Geometry check sheet. Reference: the model listing, model coordinates, mm. A direction names the side the tool comes from. Give positions to 0.01 mm unless a question says otherwise; leave off trailing zeros. Write each loop counter-clockwise with the first axis right and the second up, starting at its lowest first coordinate (ties: lowest second). Pieces come first, ordered by that corner, then holes. Notation, with made-up numbers: (87, 3.5) - (132, 3.5) arc R22 ccw to (132, 28.5) - close; hole circle Ø5 at (5, -21). An arc over 180 degrees is marked (long way). One line per question, with ' | ' between items. Start each with the question number.
Q1. Section check D-D on y = 30. Record the boundary of the cut face in (x, z).
Q2. Release check for a two-part mould opening along Y. For faces 6 (the face through (104, 28, 17)), 7 (the face through (105.014, 31.636, 17.215)), 8 (the face through (1.141, 1.203, 5.916)), 9 (the face through (64, 106, 11)) record: +Y half, -Y half, draft (parallel to the pull), parting line (faces both ways), or undercut.
Q3. Thickness scan on L1, parallel to Y at x = 105.05, z = 17; L2, parallel to Y at x = 98.5, z = 11; L3, parallel to X at y = 105.1, z = 17. Record the ranges inside material, lowest first. Write a range as [from, to].
Q4. Gauge pin test, flat ends, axial feed: P1, Ø5, axis at x = 14.5, y = 45, coming from the +Z side; P2, Ø9.5, axis at x = 86.5, z = 7, coming from the +Y side; P3, Ø1.6, axis at x = 103, y = 82.5, coming from the +Z side. Record the tip position at first contact, or that the pin passes through.
Q5. Section check A-A on x = 64. Record the boundary of the cut face in (y, z), and give its area (3 significant figures).
Q6. Section check C-C on z = 17. Record the boundary of the cut face in (x, y), and give its area (3 significant figures).
Q7. Set-up check for faces 1 (the face through (51, 53, 2)), 2 (the face through (102.797, 1.141, 5.916)), 3 (the face through (62, 104, 17)), 4 (the face through (62.536, 105.014, 17.761)), 5 (the face through (28, 104, 6)): record each of +Z, -Z, +X, -X, +Y, -Y from which the full face is reachable in a straight line by a thin tool's end or side.
Q8. Section check B-B on x = 26.5. Record the boundary of the cut face in (y, z), and give its area (3 significant figures).
```python
from build123d import *

# Parameters (mm, degrees)
EXTRUDE_2_DEPTH     = 2
EXTRUDE_3_DEPTH     = 10
SKETCH_5_W          = 7
SKETCH_5_H          = 25
CUT_EXTRUDE_1_DEPTH = 10
SKETCH_6_W          = 74
SKETCH_6_H          = 15
CUT_EXTRUDE_2_DEPTH = 10
SKETCH_7_W          = 20
SKETCH_7_H          = 2
SKETCH_7_W_2        = 2
SKETCH_7_H_2        = 20
EXTRUDE_4_DEPTH     = 22
SKETCH_8_R          = 1.65
CUT_EXTRUDE_3_DEPTH = 22
SKETCH_10_R         = 1.65
CUT_EXTRUDE_4_DEPTH = 22
FILLET_1_R          = 2


with BuildPart() as part:
    # 草图1 → 凸台-拉伸2 (new body)
    with BuildSketch(Plane.XY):
        with BuildLine():
            Line((4, 0), (100, 0))
            ThreePointArc((100, 0), (102.828427125, 1.171572875), (104, 4))
            Line((104, 4), (104, 100))
            ThreePointArc((104, 100), (102.828427125, 102.828427125), (100, 104))
            Line((100, 104), (4, 104))
            ThreePointArc((4, 104), (1.171572875, 102.828427125), (0, 100))
            Line((0, 100), (0, 4))
            ThreePointArc((0, 4), (1.171572875, 1.171572875), (4, 0))
        make_face()
    extrude(amount=EXTRUDE_2_DEPTH)

    # 草图4 → 凸台-拉伸3 (add)
    with BuildSketch(Plane.XY.offset(2)):
        with BuildLine():
            Line((104, 4), (104, 100))
            ThreePointArc((104, 100), (102.828427125, 102.828427125), (100, 104))
            Line((100, 104), (4, 104))
            ThreePointArc((4, 104), (1.171572875, 102.828427125), (0, 100))
            Line((0, 100), (0, 4))
            ThreePointArc((0, 4), (1.171572875, 1.171572875), (4, 0))
            Line((4, 0), (100, 0))
            ThreePointArc((100, 0), (102.828427125, 1.171572875), (104, 4))
        make_face()
        with BuildLine():
            Line((102, 4), (102, 100))
            ThreePointArc((102, 100), (101.414213562, 101.414213562), (100, 102))
            Line((100, 102), (4, 102))
            ThreePointArc((4, 102), (2.585786438, 101.414213562), (2, 100))
            Line((2, 100), (2, 4))
            ThreePointArc((2, 4), (2.585786438, 2.585786438), (4, 2))
            Line((4, 2), (100, 2))
            ThreePointArc((100, 2), (101.414213562, 2.585786438), (102, 4))
        make_face(mode=Mode.SUBTRACT)
    extrude(amount=EXTRUDE_3_DEPTH)

    # 草图5 → 切除-拉伸1 (cut)
    with BuildSketch(Plane(origin=(104, 0, 0), x_dir=(0, 0, -1), z_dir=(1, 0, 0))):
        with Locations((-8.5, 77.5)):
            Rectangle(SKETCH_5_W, SKETCH_5_H)
    extrude(amount=-CUT_EXTRUDE_1_DEPTH, mode=Mode.SUBTRACT)

    # 草图6 → 切除-拉伸2 (cut)
    with BuildSketch(Plane(origin=(0, 0, 0), x_dir=(-1, 0, 0), z_dir=(0, 0, -1))):
        with Locations((-52, 76.5)):
            Rectangle(SKETCH_6_W, SKETCH_6_H)
    extrude(amount=-CUT_EXTRUDE_2_DEPTH, mode=Mode.SUBTRACT)

    # 草图7 → 凸台-拉伸4 (add)
    with BuildSketch(Plane(origin=(0, 0, 0), x_dir=(-1, 0, 0), z_dir=(0, 0, -1))):
        with Locations((-64, 105)):
            Rectangle(SKETCH_7_W, SKETCH_7_H)
        with Locations((-105, 30)):
            Rectangle(SKETCH_7_W_2, SKETCH_7_H_2)
    extrude(amount=-EXTRUDE_4_DEPTH)

    # 草图8 → 切除-拉伸3 (cut)
    with BuildSketch(Plane(origin=(106, 0, 0), x_dir=(0, 0, -1), z_dir=(1, 0, 0))):
        with Locations((-17, 30)):
            Circle(SKETCH_8_R)
    extrude(amount=-CUT_EXTRUDE_3_DEPTH, mode=Mode.SUBTRACT)

    # 草图10 → 切除-拉伸4 (cut)
    with BuildSketch(Plane(origin=(0, 106, 0), x_dir=(1, 0, 0), z_dir=(0, 1, 0))):
        with Locations(Location((64, -17, 0), (0, 0, 270))):
            Circle(SKETCH_10_R)
    extrude(amount=-CUT_EXTRUDE_4_DEPTH, mode=Mode.SUBTRACT)

    # 圆角1
    fillet_1_edges = [part.edges().sort_by_distance(p)[0] for p in [
        (54, 104, 6),
        (74, 104, 6),
        (104, 40, 6),
        (104, 20, 6),
    ]]
    fillet(fillet_1_edges, radius=FILLET_1_R - 0.0001)  # a hair under: the kernel refuses the full size


solid = part.part
```
Working result:
1) outline: (0, 0) - (106, 0) - (106, 15.35) - (104, 15.35) - (104, 12) - (102, 12) - (102, 2) - (2, 2) - (2, 12) - (0, 12) - close; (104, 18.65) - (106, 18.65) - (106, 22) - (104, 22) - close
2) face 6: draft | face 7: undercut | face 8: -Y half | face 9: +Y half
3) L1: y = [20, 28.35], [31.65, 40] | L2: y = [0, 2], [102, 104] | L3: x = [54, 62.35], [65.65, 74]
4) P1: stops at z = 2 | P2: stops at y = 104 | P3: stops at z = 5
5) outline: (0, 0) - (69, 0) - (69, 2) - (2, 2) - (2, 12) - (0, 12) - close; (84, 0) - (106, 0) - (106, 15.35) - (104, 15.35) - (104, 12) - (102, 12) - (102, 2) - (84, 2) - close; (104, 18.65) - (106, 18.65) - (106, 22) - (104, 22) - close | area: 255 mm2
6) outline: (54, 104) - (62.35, 104) - (62.35, 106) - (54, 106) - close; (65.65, 104) - (74, 104) - (74, 106) - (65.65, 106) - close; (104, 20) - (106, 20) - (106, 28.35) - (104, 28.35) - close; (104, 31.65) - (106, 31.65) - (106, 40) - (104, 40) - close | area: 66.8 mm2
7) face 1: +Z | face 2: +Z, -Z, +X, -Y | face 3: +Z, +X, -X, -Y | face 4: +Y, -Y | face 5: +Z, -Z, -X, +Y
8) outline: (0, 0) - (69, 0) - (69, 2) - (2, 2) - (2, 12) - (0, 12) - close; (84, 0) - (104, 0) - (104, 12) - (102, 12) - (102, 2) - (84, 2) - close | area: 218 mm2
